The model under review builds one solid part; all positions refer to its coordinate system, in mm. Give positions to 0.01 mm unless a question says otherwise; leave off trailing zeros. Loops run counter-clockwise (first coordinate to the right, second up) from the corner with the lowest first, then second, coordinate; pieces in that order, holes last. Notation, with made-up numbers: (-12.5, 23.5) -> (46.5, 23.5) arc R24 ccw to (46.5, 48.5) -> close; hole circle Ø11 at (-28, 82.25). An arc over 180 degrees is marked (long way). Write each question's results on one line, items separated by ' | '. Start each with the question number.
Q1. We need section B-B (z = 49.5). Write out the cut boundary in (x, y), plus the area to 3 significant figures.
Q2. We need section C-C (x = 4.5). Give the number of separate pieces and of enclosed holes in the cut face, plus the area to 3 significant figures.
Q3. We need section D-D (z = 4.5). Write out the cut boundary in (x, y).
Q4. We need section A-A (z = 130). Write out the cut boundary in (x, y).
Q5. Wall thickness on L1, parallel to Z at x = 0.55, y = -4.5; L2, parallel to Y at x = 6.5, z = 88; L3, parallel to X at y = -6.5, z = 97: over which ranges is each line inside the solid? List them lowest first. Write a range as [from, to].
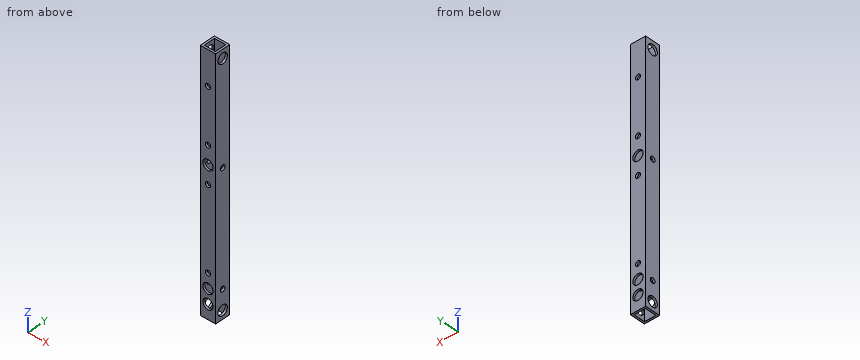
Autodesk Inventor part; units mm, degrees
ref_plane "YZ Plane" through (0, 0, 0) normal (1, 0, 0) x (0, 1, 0)
ref_plane "XZ Plane" through (0, 0, 0) normal (0, 1, 0) x (-1, 0, 0)
ref_plane "XY Plane" through (0, 0, 0) normal (0, 0, 1) x (1, 0, 0)
sketch "スケッチ1" plane through (0, 0, 0) normal (0, 0, 1) x (1, 0, 0)
  line L0 (0, 0) -> (9, 0)
  line L1 (9, 0) -> (9, -9)
  line L2 (9, -9) -> (0, -9)
  line L3 (0, -9) -> (0, 0)
  line L4 (1.2, -1.2) -> (7.8, -1.2)
  line L5 (7.8, -1.2) -> (7.8, -7.8)
  line L6 (7.8, -7.8) -> (1.2, -7.8)
  line L7 (1.2, -7.8) -> (1.2, -1.2)
  dimension "d0" = 9
  dimension "d1" = 9
  dimension "d2" = 6.6
  dimension "d3" = 6.6
  dimension "d4" = 1.2
  dimension "d5" = 1.2
extrude "押し出し1" add sketch "スケッチ1" along normal blind 75
sketch "スケッチ2" plane through (9, -9, 0) normal (1, 0, 0) x (0, 0, -1)
  line L0 (0, 9) -> (-75, 9)
  line L1 (0, 0) -> (0, 9)
  line L2 (-75, 0) -> (-75, 9)
  point P0 (-70.5, 4.5)
  point P1 (-4.5, 4.5)
  dimension "d8" = 4.5
  dimension "d9" = 4.5
  dimension "d10" = 4.5
  dimension "d11" = 4.5
hole "穴1" at (9, -4.5, 70.5) at (9, -4.5, 4.5) direction (-1, 0, 0) diameter 3 end through all
sketch "スケッチ3" plane through (0, 0, 0) normal (0, 1, 0) x (1, 0, 0)
  line L0 (0, 0) -> (0, -75)
  line L1 (9, 0) -> (0, 0)
  line L2 (9, -75) -> (0, -75)
  point P0 (4.5, -61.5)
  point P1 (4.5, -13.5)
  dimension "d19" = 4.5
  dimension "d20" = 4.5
  dimension "d21" = 13.5
  dimension "d22" = 13.5
hole "穴2" at (4.5, 0, 61.5) at (4.5, 0, 13.5) direction (0, -1, 0) diameter 3 end through all
sketch "スケッチ6" plane through (0, 0, 75) normal (0, 0, 1) x (1, 0, 0)
  line L0 (0, -9) -> (9, -9)
  line L1 (0, 0) -> (9, 0)
  line L2 (9, 0) -> (9, -9)
  line L3 (9, -9) -> (0, -9)
  line L4 (0, -9) -> (0, 0)
  line L5 (1.2, -1.2) -> (7.8, -1.2)
  line L6 (7.8, -1.2) -> (7.8, -7.8)
  line L7 (1.2, -1.2) -> (7.8, -1.2)
  line L8 (7.8, -1.2) -> (7.8, -7.8)
  line L9 (7.8, -7.8) -> (1.2, -7.8)
  line L10 (1.2, -7.8) -> (1.2, -1.2)
extrude "押し出し3" add sketch "スケッチ6" along normal blind 60
sketch "スケッチ7" plane through (9, -9, 0) normal (1, 0, 0) x (0, 0, -1)
  line L0 (-135, 0) -> (-135, 9)
  line L1 (0, 9) -> (-135, 9)
  point P0 (-130, 4.5)
  dimension "d43" = 5
  dimension "d44" = 4.5
hole "穴4" at (9, -4.5, 130) direction (-1, 0, 0) diameter 6 end through all
sketch "スケッチ8" plane through (0, 0, 0) normal (0, 0, -1) x (-1, 0, 0)
  line L0 (-9, -9) -> (-9, 0)
  line L1 (0, 0) -> (-9, 0)
  line L2 (-9, 0) -> (-9, -9)
  line L3 (-9, -9) -> (0, -9)
  line L4 (0, -9) -> (0, 0)
  line L5 (-7.8, -7.8) -> (-1.2, -7.8)
  line L6 (-7.8, -7.8) -> (-1.2, -7.8)
  line L7 (-1.2, -7.8) -> (-1.2, -1.2)
  line L8 (-1.2, -1.2) -> (-7.8, -1.2)
  line L9 (-7.8, -1.2) -> (-7.8, -7.8)
extrude "押し出し4" add sketch "スケッチ8" along normal blind 12
sketch "スケッチ9" plane through (0, -9, 135) normal (-1, 0, 0) x (0, 0, 1)
  line L0 (-147, 0) -> (-147, 9)
  line L1 (0, 0) -> (-147, 0)
  point P0 (-135, 9)
  point P1 (-142, 4.5)
  dimension "d54" = 5
  dimension "d55" = 4.5
hole "穴5" at (0, -4.5, -7) direction (1, 0, 0) diameter 6 end through all
sketch "スケッチ10" plane through (0, -9, 135) normal (0, -1, 0) x (1, 0, 0)
  line L0 (0, 0) -> (9, 0)
  line L1 (0, 0) -> (0, -147)
  point P0 (0, -135)
  point P1 (4.5, -52)
  point P2 (4.5, -20)
  dimension "d63" = 20
  dimension "d64" = 32
  dimension "d65" = 4.5
  dimension "d66" = 4.5
hole "穴6" at (4.5, -9, 83) at (4.5, -9, 115) direction (0, 1, 0) diameter 3 end through all
sketch "スケッチ11" plane through (0, -9, 135) normal (-1, 0, 0) x (0, 0, 1)
  point P0 (-135, 9)
sketch "スケッチ12" plane through (0, 0, 135) normal (0, 1, 0) x (1, 0, 0)
  line L0 (0, 147) -> (0, 0)
  line L1 (0, 147) -> (9, 147)
  circle A0 centre (4.5, 121.5) radius 1.5
  point P0 (0, 135)
  point P1 (4.5, 138.5)
  point P2 (4.5, 130)
  dimension "d74" = 4.5
  dimension "d75" = 25.5
  dimension "d76" = 8.5
  dimension "d77" = 8.5
  dimension "d78" = 4.5
hole "穴7" at (4.5, 0, 5) at (4.5, 0, -3.5) direction (0, -1, 0) diameter 6 end through all
sketch "スケッチ13" plane through (0, 0, 135) normal (0, 1, 0) x (1, 0, 0)
  circle A0 centre (4.5, 52) radius 1.5
  circle A1 centre (4.5, 73.5) radius 1.5
  line L0 (0, 147) -> (0, 0)
  point P0 (0, 135)
  point P1 (4.5, 62.75)
  dimension "d86" = 21.5
  dimension "d87" = 10.75
  dimension "d88" = 4.5
hole "穴8" at (4.5, 0, 72.25) direction (0, -1, 0) diameter 6 end through all
properties part number "上下直動9x9_3" material "アルミニウム 6061"
Output:
1) outline: (0, -9) -> (9, -9) -> (9, 0) -> (0, 0) -> close; hole (1.2, -7.8) -> (7.8, -7.8) -> (7.8, -1.2) -> (1.2, -1.2) -> close | area: 37.4 mm2
2) separate pieces: 16 | enclosed holes: 0 | area: 281 mm2
3) outline: (0, -9) -> (1.54, -9) -> (1.54, -7.8) -> (1.2, -7.8) -> (1.2, -6) -> (0, -6) -> close; (0, -3) -> (1.2, -3) -> (1.2, -1.2) -> (1.54, -1.2) -> (1.54, 0) -> (0, 0) -> close; (7.46, -9) -> (9, -9) -> (9, -6) -> (7.8, -6) -> (7.8, -7.8) -> (7.46, -7.8) -> close; (7.46, -1.2) -> (7.8, -1.2) -> (7.8, -3) -> (9, -3) -> (9, 0) -> (7.46, 0) -> close
4) outline: (0, -9) -> (9, -9) -> (9, -7.5) -> (7.8, -7.5) -> (7.8, -7.8) -> (1.2, -7.8) -> (1.2, -7.5) -> (0, -7.5) -> close; (0, -1.5) -> (1.2, -1.5) -> (1.2, -1.2) -> (7.8, -1.2) -> (7.8, -1.5) -> (9, -1.5) -> (9, 0) -> (0, 0) -> close
5) L1: [-12, -10], [-4, 3], [6, 69], [72, 127], [133, 135] | L2: [-9, -7.8], [-1.2, 0] | L3: [0, 1.2], [7.8, 9]
